Read the model definition and answer for the solid it produces. Units are mm, in the model's axes. Coordinates: 2 decimals unless noted, no trailing zeros. Return JSON: item names as keys, results as strings.
Autodesk Inventor part; units mm, degrees
ref_plane "YZ Plane" through (0, 0, 0) normal (1, 0, 0) x (0, 1, 0)
ref_plane "XZ Plane" through (0, 0, 0) normal (0, 1, 0) x (-1, 0, 0)
ref_plane "XY Plane" through (0, 0, 0) normal (0, 0, 1) x (1, 0, 0)
sketch "Skizze1" plane through (0, 0, 0) normal (0, 1, 0) x (-1, 0, 0)
  line L0 (0, 0) -> (-710, 0)
  line L1 (-710, 0) -> (-710, 597)
  line L2 (-710, 597) -> (0, 597)
  line L3 (0, 597) -> (0, 0)
  line L4 (-355, 0) -> (-355, 597) construction
  line L5 (0, 298.5) -> (-710, 298.5) construction
  line L6 (-190, 0) -> (-190, 597) construction
  line L7 (-520, 0) -> (-520, 597) construction
  line L8 (-710, 407) -> (0, 407) construction
  line L9 (0, 80) -> (-710, 80) construction
  line L10 (-695, 582) -> (-695, 15) construction
  line L11 (-695, 15) -> (-15, 15) construction
  line L12 (-15, 15) -> (-15, 582) construction
  line L13 (-15, 582) -> (-695, 582) construction
  line L14 (-23, 362) -> (-7, 362) construction
  line L15 (-7, 362) -> (-7, 452) construction
  line L16 (-7, 452) -> (-23, 452) construction
  line L17 (-23, 452) -> (-23, 362) construction
  line L18 (-23, 362) -> (-7, 452) construction
  line L19 (-7, 362) -> (-23, 452) construction
  line L20 (-142.5, 590) -> (-237.5, 590) construction
  line L21 (-237.5, 590) -> (-237.5, 574) construction
  line L22 (-237.5, 574) -> (-142.5, 574) construction
  line L23 (-142.5, 574) -> (-142.5, 590) construction
  line L24 (-142.5, 590) -> (-237.5, 574) construction
  line L25 (-237.5, 590) -> (-142.5, 574) construction
  line L26 (-307.5, 590) -> (-402.5, 590) construction
  line L27 (-402.5, 590) -> (-402.5, 574) construction
  line L28 (-402.5, 574) -> (-307.5, 574) construction
  line L29 (-307.5, 574) -> (-307.5, 590) construction
  line L30 (-307.5, 590) -> (-402.5, 574) construction
  line L31 (-402.5, 590) -> (-307.5, 574) construction
  circle A0 centre (-15, 399.5) radius 3.25
  circle A1 centre (-15, 370) radius 4.5
  circle A2 centre (-15, 414.5) radius 3.25
  circle A3 centre (-15, 444) radius 4.5
  circle A4 centre (-182.5, 582) radius 3.25
  circle A5 centre (-153, 582) radius 4.5
  circle A6 centre (-318, 582) radius 4.5
  circle A7 centre (-347.5, 582) radius 3.25
  circle A8 centre (-197.5, 582) radius 3.25
  circle A9 centre (-227, 582) radius 4.5
  circle A10 centre (-392, 582) radius 4.5
  circle A11 centre (-362.5, 582) radius 3.25
  circle A12 centre (-695, 399.5) radius 3.25
  circle A13 centre (-695, 370) radius 4.5
  circle A14 centre (-695, 444) radius 4.5
  circle A15 centre (-695, 414.5) radius 3.25
  circle A16 centre (-527.5, 582) radius 3.25
  circle A17 centre (-557, 582) radius 4.5
  circle A18 centre (-512.5, 582) radius 3.25
  circle A19 centre (-483, 582) radius 4.5
  circle A20 centre (-15, 43) radius 4.5
  circle A21 centre (-15, 72.5) radius 3.25
  circle A22 centre (-190, 238.5) radius 2.75
  circle A23 centre (-190, 358.5) radius 2.75
  circle A24 centre (-520, 238.5) radius 2.75
  circle A25 centre (-520, 358.5) radius 2.75
  circle A26 centre (-15, 117) radius 4.5
  circle A27 centre (-15, 87.5) radius 3.25
  circle A28 centre (-695, 43) radius 4.5
  circle A29 centre (-695, 72.5) radius 3.25
  circle A30 centre (-695, 87.5) radius 3.25
  circle A31 centre (-695, 117) radius 4.5
  line L32 (-115, 597) -> (-115, 562)
  line L33 (-115, 562) -> (-35, 482)
  line L34 (-35, 482) -> (0, 482)
  line L35 (-595, 597) -> (-595, 562)
  line L36 (-595, 562) -> (-675, 482)
  line L37 (-675, 482) -> (-710, 482)
  point P0 (-15, 407)
  point P1 (-190, 582)
  point P2 (-355, 582)
  point P3 (-190, 298.5)
  dimension "d0" = 710
  dimension "d1" = 597
  dimension "d2" = 190
  dimension "d3" = 80
  dimension "d4" = 190
  dimension "d5" = 190
  dimension "d6" = 15
  dimension "d7" = 16
  dimension "d8" = 90
  dimension "d9" = 95
  dimension "d10" = 16
  dimension "d11" = 95
  dimension "d12" = 16
  dimension "d13" = 6.5
  dimension "d14" = 7.5
  dimension "d15" = 9
  dimension "d16" = 37
  dimension "d17" = 6.5
  dimension "d18" = 9
  dimension "d19" = 7.5
  dimension "d20" = 37
  dimension "d21" = 6.5
  dimension "d22" = 9
  dimension "d23" = 7.5
  dimension "d24" = 37
  dimension "d30" = 5.5
  dimension "d31" = 60
  dimension "d34" = 6.5
  dimension "d35" = 9
  dimension "d36" = 7.5
  dimension "d37" = 37
  dimension "d80" = 680
  dimension "d81" = 45
  dimension "d83" = 115
  dimension "d84" = 115
  dimension "d85" = 35
extrude "Ex-Platte" add sketch "Skizze1" along normal blind 3 contours L0 L1 L37 L36 L35 L2 L32 L33 L34 L3
chamfer "Fase-15mm" distance 15 angle 45 6 edges at (710, 1.5, 0) (0, 1.5, 0) (0, 1.5, 482) (115, 1.5, 597) (595, 1.5, 597) (710, 1.5, 482)
sketch "Profil-Verstärkung" plane through (0, 0, 0) normal (0, 1, 0) x (-1, 0, 0)
  line L0 (-695, 0) -> (-15, 0)
  line L1 (0, 15) -> (0, 482)
  line L2 (-115, 597) -> (-595, 597)
  line L3 (-710, 482) -> (-710, 15)
  line L4 (0, 298.5) -> (-710, 298.5) construction
  circle A0 centre (-15, 117) radius 4.5
  circle A1 centre (-15, 370) radius 4.5
  circle A2 centre (-190, 358.5) radius 2.75
  circle A3 centre (-190, 238.5) radius 2.75
  circle A4 centre (-227, 582) radius 4.5
  circle A5 centre (-318, 582) radius 4.5
  line L5 (-355, 0) -> (-355, 597) construction
  circle A6 centre (-355, 298.5) radius 2.5
  circle A7 centre (-435, 298.5) radius 2.5
  circle A8 centre (-515, 298.5) radius 2.5
  circle A9 centre (-595, 298.5) radius 2.5
  circle A10 centre (-675, 298.5) radius 2.5
  circle A11 centre (-355, 323.5) radius 2.5
  circle A12 centre (-355, 403.5) radius 2.5
  circle A13 centre (-355, 483.5) radius 2.5
  circle A14 centre (-355, 563.5) radius 2.5
  circle A15 centre (-275, 298.5) radius 2.5
  circle A16 centre (-195, 298.5) radius 2.5
  circle A17 centre (-115, 298.5) radius 2.5
  circle A18 centre (-35, 298.5) radius 2.5
  circle A19 centre (-355, 273.5) radius 2.5
  circle A20 centre (-355, 193.5) radius 2.5
  circle A21 centre (-355, 113.5) radius 2.5
  circle A22 centre (-355, 33.5) radius 2.5
  point P0 (0, 0)
  point P1 (0, 582)
  point P2 (-15, 597)
  point P3 (-695, 597)
  point P4 (-710, 582)
  dimension "d38" = 710
  dimension "d40" = 121.5
  dimension "d42" = 11.5
  dimension "d61" = 5
  dimension "d64" = 80
  dimension "d69" = 5
  dimension "d70" = 25
  dimension "d73" = 80
extrude "Ex-ProfilBohrungen" cut sketch "Profil-Verstärkung" along normal up to surface (3 mm away) contours A6 | A7 | A8 | A9 | A10 | A11 | A12 | A13 | A14 | A15 | A16 | A17 | A18 | A19 | A20 | A21 | A22
equation "\"d5\" = d4"
equation "\"d17\" = d13"
equation "\"d18\" = d15"
equation "\"d19\" = d14"
equation "\"d20\" = d16"
equation "\"d21\" = d13"
equation "\"d22\" = d15"
equation "\"d23\" = d14"
equation "\"d24\" = d16"
equation "\"d34\" = d13"
equation "\"d35\" = d15"
equation "\"d36\" = d14"
equation "\"d37\" = d16"
equation "\"d84\" = d83"
equation "\"d69\" = d61"
properties part number "enc-FrontPanel Unten"
1. Consider L1, parallel to X at y = 1.7, z = 238.5; L2, parallel to X at y = 0.45, z = 445; L3, parallel to Z at x = 190, y = 2.1. Determine where each line is inside the solid, lowest interval first.
Taken from the geometry:
{"L1": "x = 0 to 187.25, 192.75 to 517.25, 522.75 to 710", "L2": "x = 0 to 10.61, 19.39 to 690.61, 699.39 to 710", "L3": "z = 0 to 235.75, 241.25 to 355.75, 361.25 to 597"}
2. Flat-ended cylindrical pins translate along their axes: pin 1 Ø3 at (x, z) = (515, 298.5) entering from +Y; pin 2 Ø6 at (x, z) = (588, 299) entering from -Y; pin 3 Ø0.9 at (x, y) = (25, 2) entering from +Z. Find the tip coordinate at first contact, or state that the pin passes through.
Taken from the geometry:
{"pin 1": "passes through", "pin 2": "stops at y = 0", "pin 3": "stops at z = 482"}
3. The part is cut by section A-A (y = 2.55). Count the separate pieces of the cut face and the enclosed holes in it, then the cut area to 3 significant figures.
Taken from the geometry:
{"separate pieces": "1", "enclosed holes": "49", "area": "401,000 mm2"}
